Job drawing, mm, ordinate dimensions from the low corner. One solid piece. A direction names the side the tool comes from. Give positions to 0.01 mm unless a question says otherwise; leave off trailing zeros. Order: outer loops, then holes, each group sorted by start corner. A loop starts at its lowest first (then second) coordinate and runs counter-clockwise, first axis right, second up.
Item 1: Which spindle directions (+Z, -Z, +X, -X, +Y, -Y) get a long thin tool onto all of the face, cutting with end or side? Do the marked faces 1 and 2. Say none if no direction does.
Item 2: Band-saw the part on A-A on x = 2.9. Give the cut face in (y, z), plus the area to 3 significant figures.
Item 3: Flat gauge pins, fed straight in: P1, Ø0.8, axis at y = 3.5, z = 1, coming from the -X side; P2, Ø1, axis at x = 2, z = 15.5, coming from the -Y side; P3, Ø3, axis at y = 5, z = 8, coming from the -X side. Where does each tip first touch, or does it go through?
Item 4: Wall check: L1, parallel to Z at x = 3.55, y = 2.45; L2, parallel to Y at x = 2.95, z = 13; L3, parallel to Y at x = 2.25, z = 1.25. Give the ranges that are in metal, low to high.
Item 5: Band-saw the part on C-C on z = 17.25. Give the cut face in (x, y).
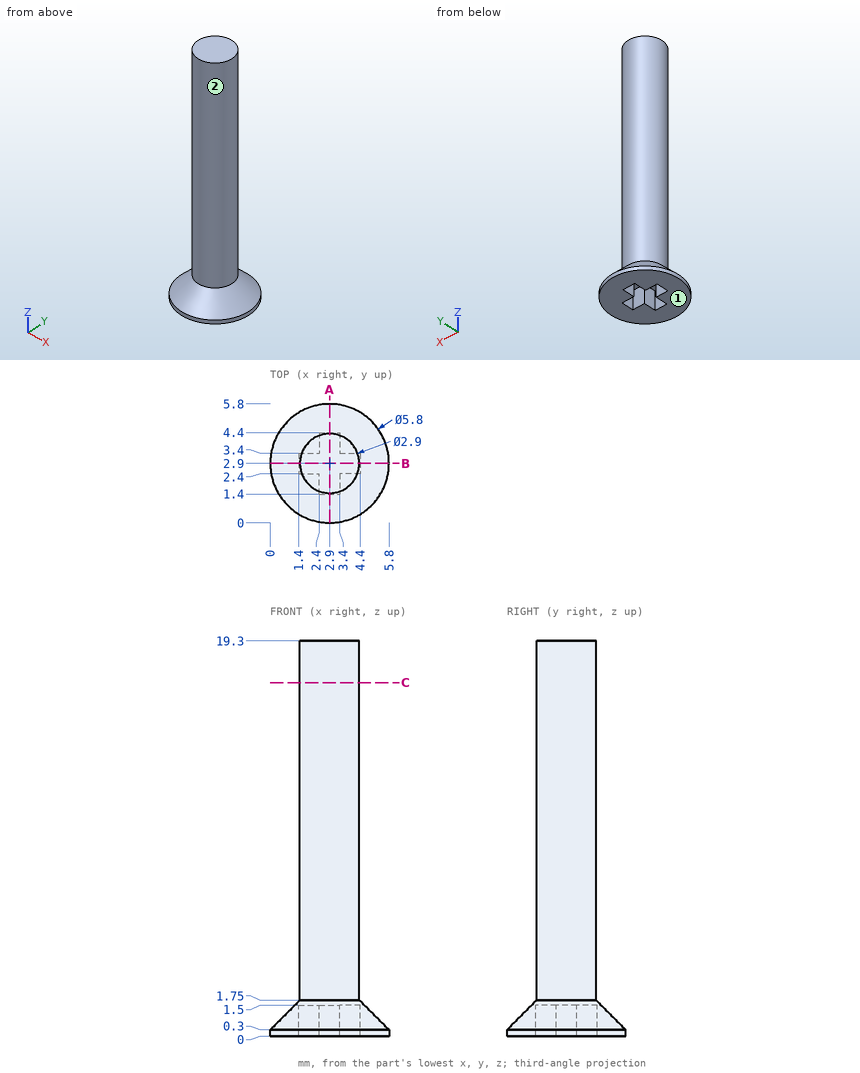
The answers:
1. face 1: -Z, +X, -X, +Y, -Y
1. face 2: +Z
2. outline: (0, 0) - (1.4, 0) - (1.4, 1.5) - (4.4, 1.5) - (4.4, 0) - (5.8, 0) - (5.8, 0.3) - (4.35, 1.75) - (4.35, 19.3) - (1.45, 19.3) - (1.45, 1.75) - (0, 0.3) - close
2. area: 54.4 mm2
3. P1: stops at x = 0.36
3. P2: stops at y = 1.51
3. P3: stops at x = 1.58
4. L1: z = 1.5 to 19.3
4. L2: y = 1.45 to 4.35
4. L3: y = 1.06 to 2.4, 3.4 to 4.74
5. outline: circle Ø2.9 at (2.9, 2.9)
